from build123d import *

# Parameters (mm, degrees)
SKETCH1_R           = 0.875
SKETCH1_R_2         = 3.5
BOSS_EXTRUDE1_DEPTH = 3
BOSS_EXTRUDE2_START = -2
SKETCH2_R           = 3.5
BOSS_EXTRUDE2_DEPTH = 2
FILLET1_R           = 0.25


with BuildPart() as part:
    # Sketch1 → Boss-Extrude1 (new body)
    with BuildSketch(Plane(origin=(0, 8.778505218, 0), x_dir=(1, 0, 0), z_dir=(0, 1, 0))):
        with BuildLine():
            Line((39.666515042, -34.709383283), (12.072408659, -37.266851361))
            ThreePointArc((12.072408659, -37.266851361), (10.483909442, -39.009383283), (12.072408659, -40.751915204))
            Line((12.072408659, -40.751915204), (39.666515042, -43.309383283))
            ThreePointArc((39.666515042, -43.309383283), (43.483909442, -44.759383283), (47.301303841, -43.309383283))
            Line((47.301303841, -43.309383283), (60.330539136, -41.485236238))
            ThreePointArc((60.330539136, -41.485236238), (62.483909442, -39.009383283), (60.330539136, -36.533530328))
            Line((60.330539136, -36.533530328), (47.301303841, -34.709383283))
            ThreePointArc((47.301303841, -34.709383283), (43.483909442, -33.259383283), (39.666515042, -34.709383283))
        make_face()
        with Locations(Location((27.233909442, -39.009383283, 0), (0, 0, 270))):
            Circle(SKETCH1_R, mode=Mode.SUBTRACT)
        with Locations(Location((30.233909442, -39.009383283, 0), (0, 0, 270))):
            Circle(SKETCH1_R, mode=Mode.SUBTRACT)
        with Locations(Location((33.233909442, -39.009383283, 0), (0, 0, 270))):
            Circle(SKETCH1_R, mode=Mode.SUBTRACT)
        with Locations(Location((36.233909442, -39.009383283, 0), (0, 0, 270))):
            Circle(SKETCH1_R, mode=Mode.SUBTRACT)
        with Locations(Location((43.483909442, -39.009383283, 0), (0, 0, 270))):
            Circle(SKETCH1_R_2, mode=Mode.SUBTRACT)
        with Locations(Location((50.733909442, -39.009383283, 0), (0, 0, 270))):
            Circle(SKETCH1_R, mode=Mode.SUBTRACT)
        with Locations(Location((53.733909442, -39.009383283, 0), (0, 0, 270))):
            Circle(SKETCH1_R, mode=Mode.SUBTRACT)
        with Locations(Location((56.733909442, -39.009383283, 0), (0, 0, 270))):
            Circle(SKETCH1_R, mode=Mode.SUBTRACT)
        with Locations(Location((59.733909442, -39.009383283, 0), (0, 0, 270))):
            Circle(SKETCH1_R, mode=Mode.SUBTRACT)
    extrude(amount=BOSS_EXTRUDE1_DEPTH)

    # Sketch2 → Boss-Extrude2 (add)
    with BuildSketch(Plane(origin=(0, 11.778505218, 0), x_dir=(1, 0, 0), z_dir=(0, 1, 0)).offset(BOSS_EXTRUDE2_START)):
        with Locations(Location((43.483909442, -39.009383283, 0), (0, 0, 270))):
            Circle(SKETCH2_R)
    extrude(amount=BOSS_EXTRUDE2_DEPTH)

    # Fillet1
    fillet1_edges = [part.edges().sort_by_distance(p)[0] for p in [
        (25.869461851, 11.778505218, 42.030649244),
        (43.483909442, 11.778505218, 44.759383283),
        (53.815921489, 11.778505218, 42.39730976),
        (62.483909442, 11.778505218, 39.009383283),
        (53.815921489, 11.778505218, 35.621456805),
        (43.483909442, 11.778505218, 33.259383283),
        (25.869461851, 11.778505218, 35.988117322),
        (10.483909442, 11.778505218, 39.009383283),
    ]]
    fillet(fillet1_edges, radius=FILLET1_R)


solid = part.part
Check sheet for the modelled part. Datum: model origin and axes. Units: mm. Coordinates: 2 decimals unless noted, no trailing zeros.
Item 1: Depth check by flat-ended pin: pin 1 Ø2 at (x, z) = (45, 38) entering from -Y. Enter the tip coordinate at first touch or a pass-through.
Numbers:
pin 1: stops at y = 9.78
Item 2: Scan lines: probe 1 along Z at (x, y) = (49, 11.4); probe 2 along Z at (x, y) = (57, 10.2); probe 3 along X at (y, z) = (9.3, 37.5). Record each from-to range of solid material in increasing order.
Numbers:
probe 1: z = 34.95 to 43.07
probe 2: z = 36.07 to 38.18, 39.84 to 41.95
probe 3: x = 11.35 to 40.33, 46.64 to 61.98
Item 3: Cross-section at A-A on y = 9.3. Count the separate pieces of the cut face and the enclosed holes in it, then the cut area to 3 significant figures.
Numbers:
separate pieces: 1
enclosed holes: 9
area: 290 mm2
Item 4: Mould release check, pull along X, two halves, no side actions. Record for faces 1 (the face through (10.484, 10.134, 38.973)), 2 (the face through (56.772, 10.258, 38.135)), 3 (the face through (46.435, 9.272, 40.891)), 4 (the face through (43.43, 10.13, 44.76)): released by +X, released by -X, zero draft, split by the parting line, or undercut.
Numbers:
face 1: released by -X
face 2: undercut
face 3: undercut
face 4: split by the parting line
